from build123d import *

# Parameters (mm, degrees)
SKETCH1_W                = 12.7
SKETCH1_H                = 457.2
BOSS_EXTRUDE1_DEPTH      = 3.175
SKETCH2_W                = 3.175
SKETCH2_H                = 12.7
BOSS_EXTRUDE2_DEPTH      = 9.525
BOSS_EXTRUDE3_DEPTH      = 6.35
BOSS_EXTRUDE3_DEPTH_BACK = 9.525
SKETCH3_R                = 2.337311212


with BuildPart() as part:
    # Sketch1 → Boss-Extrude1 (new body)
    with BuildSketch(Plane(origin=(0, 0, 0), x_dir=(0, 0, -1), z_dir=(1, 0, 0))):
        with Locations((-4.081130849, 198.273055815)):
            Rectangle(SKETCH1_W, SKETCH1_H)
        with BuildLine():
            Line((-7.256130849, -23.976944185), (-7.256130849, 420.523055815))
            ThreePointArc((-7.256130849, 420.523055815), (-4.081130849, 423.698055815), (-0.906130849, 420.523055815))
            Line((-0.906130849, 420.523055815), (-0.906130849, -23.976944185))
            ThreePointArc((-0.906130849, -23.976944185), (-4.081130849, -27.151944185), (-7.256130849, -23.976944185))
        make_face(mode=Mode.SUBTRACT)
    extrude(amount=BOSS_EXTRUDE1_DEPTH)

    # Sketch2 → Boss-Extrude2 (add)
    with BuildSketch(Plane(origin=(0, 426.873055815, 0), x_dir=(1, 0, 0), z_dir=(0, 1, 0))):
        with Locations((1.5875, -4.081130849)):
            Rectangle(SKETCH2_W, SKETCH2_H)
    extrude(amount=BOSS_EXTRUDE2_DEPTH)

    # Sketch3 → Boss-Extrude3 (add, two sides: drawn at the far end of the back side and taken through both)
    with BuildSketch(Plane(origin=(3.175, 0, 0), x_dir=(0, 0, -1), z_dir=(1, 0, 0)).offset(-BOSS_EXTRUDE3_DEPTH_BACK)):
        with Locations((-4.081130849, 430.048055815)):
            Circle(SKETCH3_R)
    extrude(amount=BOSS_EXTRUDE3_DEPTH + BOSS_EXTRUDE3_DEPTH_BACK)


solid = part.part
Verification items for the finished model (mm, model axes). Give positions to 0.01 mm unless a question says otherwise; leave off trailing zeros. Loops run counter-clockwise (first coordinate to the right, second up) from the corner with the lowest first, then second, coordinate; pieces in that order, holes last.
1. Material ranges on probe 1 along Z at (x, y) = (0.25, 76); probe 2 along Y at (x, z) = (2, 4.75); probe 3 along Y at (x, z) = (-4, 3.75), recorded low to high.
Derived:
probe 1: z = -2.27 to 0.91, 7.26 to 10.43
probe 2: y = -30.33 to -27.08, 423.63 to 436.4
probe 3: y = 427.73 to 432.36
2. Go/stop test with flat-tipped pins: P1, Ø4, axis at x = 5, y = 32.5, coming from the -Z side; P2, Ø5, axis at x = -3.5, y = 370, coming from the +Z side; P3, Ø6.5, axis at y = 267, z = 2, coming from the -X side; P4, Ø6.5, axis at y = 229.5, z = 2.5, coming from the +X side (3 decimals). Record where each tip stops, or that it passes through.
Derived:
P1: stops at z = -2.27
P2: passes through
P3: stops at x = 0
P4: stops at x = 3.175
3. Cross-section at A-A on y = 43. Record the cut outline in (x, z) (3 decimals).
Derived:
outline: (0, -2.269) - (3.175, -2.269) - (3.175, 0.906) - (0, 0.906) - close; (0, 7.256) - (3.175, 7.256) - (3.175, 10.431) - (0, 10.431) - close
